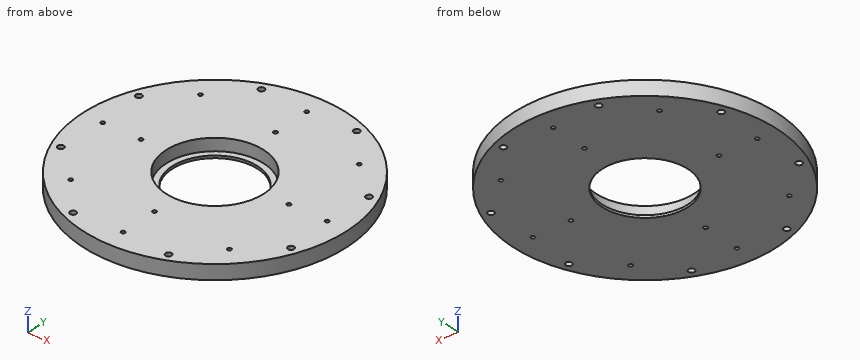
from build123d import *

# Parameters (mm, degrees)
SKETCH001_R     = 108
SKETCH001_R_2   = 35
SKETCH001_R_3   = 2.5
SKETCH001_R_4   = 1.5625
PAD_DEPTH       = 12
SKETCH_R        = 1.5625
POCKET_DEPTH    = 12.001
SKETCH002_R     = 40
POCKET001_DEPTH = 10


with BuildPart() as part:
    # Sketch001 → Pad (new body)
    with BuildSketch(Plane(origin=(0, 0, 0), x_dir=(1, 0, 0), z_dir=(0, 0, -1))):
        Circle(SKETCH001_R)
        Circle(SKETCH001_R_2, mode=Mode.SUBTRACT)
        with Locations((38.651027, 93.311833)):
            Circle(SKETCH001_R_3, mode=Mode.SUBTRACT)
        with Locations((93.311833, 38.651027)):
            Circle(SKETCH001_R_3, mode=Mode.SUBTRACT)
        with Locations((93.311833, -38.651027)):
            Circle(SKETCH001_R_3, mode=Mode.SUBTRACT)
        with Locations((38.651027, -93.311833)):
            Circle(SKETCH001_R_3, mode=Mode.SUBTRACT)
        with Locations((-38.651027, 93.311833)):
            Circle(SKETCH001_R_3, mode=Mode.SUBTRACT)
        with Locations((-93.311833, 38.651027)):
            Circle(SKETCH001_R_3, mode=Mode.SUBTRACT)
        with Locations((-93.311833, -38.651027)):
            Circle(SKETCH001_R_3, mode=Mode.SUBTRACT)
        with Locations((-38.651027, -93.311833)):
            Circle(SKETCH001_R_3, mode=Mode.SUBTRACT)
        with Locations((0, 60)):
            Circle(SKETCH001_R_4, mode=Mode.SUBTRACT)
        with Locations((-60, 0)):
            Circle(SKETCH001_R_4, mode=Mode.SUBTRACT)
        with Locations((0, -60)):
            Circle(SKETCH001_R_4, mode=Mode.SUBTRACT)
        with Locations((60, 0)):
            Circle(SKETCH001_R_4, mode=Mode.SUBTRACT)
    extrude(amount=PAD_DEPTH)

    # Sketch → Pocket (cut, through all)
    with BuildSketch(Plane.XY):
        with Locations((64.346717, 64.346717)):
            Circle(SKETCH_R)
        with Locations((0, 91)):
            Circle(SKETCH_R)
        with Locations((91, 0)):
            Circle(SKETCH_R)
        with Locations((64.346717, -64.346717)):
            Circle(SKETCH_R)
        with Locations((0, -91)):
            Circle(SKETCH_R)
        with Locations((-91, 0)):
            Circle(SKETCH_R)
        with Locations((-64.346717, -64.346717)):
            Circle(SKETCH_R)
        with Locations((-64.346717, 64.346717)):
            Circle(SKETCH_R)
    extrude(amount=-POCKET_DEPTH, mode=Mode.SUBTRACT)

    # Sketch002 (on Face2 of Pocket) → Pocket001 (cut)
    with BuildSketch(Plane.XY):
        Circle(SKETCH002_R)
    extrude(amount=-POCKET001_DEPTH, mode=Mode.SUBTRACT)


solid = part.part
Model file for the job. Use its own axes, mm. Coordinates: 2 decimals unless noted, no trailing zeros. Order: outer loops, then holes, each group sorted by start corner. A loop starts at its lowest first (then second) coordinate and runs counter-clockwise, first axis right, second up. Notation, with made-up numbers: (-13, -5.75) -> (26, -5.75) arc R14 cw to (26, 11.25) -> close; hole circle Ø6 at (8, 64). An arc over 180 degrees is marked (long way). Return JSON: item names as keys, results as strings. Group by question number.
Item 1: Saw through at B-B on z = -3.75. State how many separate pieces and enclosed holes the cut face has, then the cut area to 3 significant figures.
Item 2: Saw through at D-D on x = 73. Write the cut outline in (y, z).
Item 3: Flat gauge pins, fed straight in: P1, Ø1, axis at x = 41, z = -9.5, coming from the +Y side; P2, Ø1.5, axis at y = 41, z = -8, coming from the +X side. Where does each tip first touch, or does it go through?
Item 4: Wall check: line 1 along Y through (x, z) = (0, -3); line 2 along Y through (x, z) = (-93, -1); line 3 along X through (y, z) = (-95.5, -2). Give the ranges that are in metal, low to high. Write a range as [from, to].
Item 5: Saw through at C-C on x = 12.5. Write the cut outline in (y, z), then the cut area to 3 significant figures.
Item 6: Saw through at A-A on x = -23.5. Write the cut outline in (y, z).
Values found:
{
 "1": {"separate pieces": "1", "enclosed holes": "21", "area": "31,400 mm2"},
 "2": {"outline": "(-79.59, -12) -> (79.59, -12) -> (79.59, 0) -> (-79.59, 0) -> close"},
 "3": {"P1": "stops at y = 100.12", "P2": "stops at x = 100.22"},
 "4": {"line 1": "y = [-108, -92.56], [-89.44, -61.56], [-58.44, -40], [40, 58.44], [61.56, 89.44], [92.56, 108]", "line 2": "y = [-54.91, -41.13], [-36.17, 36.17], [41.13, 54.91]", "line 3": "x = [-50.44, -39.86], [-37.44, 37.44], [39.86, 50.44]"},
 "5": {"outline": "(-107.27, -12) -> (-32.69, -12) -> (-32.69, -10) -> (-38, -10) -> (-38, 0) -> (-107.27, 0) -> close; (32.69, -12) -> (107.27, -12) -> (107.27, 0) -> (38, 0) -> (38, -10) -> (32.69, -10) -> close", "area": "1,680 mm2"},
 "6": {"outline": "(-105.41, -12) -> (-25.94, -12) -> (-25.94, -10) -> (-32.37, -10) -> (-32.37, 0) -> (-105.41, 0) -> close; (25.94, -12) -> (105.41, -12) -> (105.41, 0) -> (32.37, 0) -> (32.37, -10) -> (25.94, -10) -> close"}
}
